For this review, take the finished solid that the model builds, in its own axes (mm). A direction names the side the tool comes from. Coordinates: 2 decimals unless noted, no trailing zeros. Loops run counter-clockwise (first coordinate to the right, second up) from the corner with the lowest first, then second, coordinate; pieces in that order, holes last. Notation, with made-up numbers: M -17,68 L 24,68 A11 cw 24,77 Z; hole C -15.75,-4 d1. An arc over 180 degrees is marked long. Put each result on its own line as item: value.
Autodesk Inventor part; units mm, degrees
ref_plane "YZ Plane" through (0, 0, 0) normal (1, 0, 0) x (0, 1, 0)
ref_plane "XZ Plane" through (0, 0, 0) normal (0, 1, 0) x (-1, 0, 0)
ref_plane "XY Plane" through (0, 0, 0) normal (0, 0, 1) x (1, 0, 0)
sketch "草图1" plane through (0, 0, 0) normal (0, 0, 1) x (1, 0, 0)
  line L0 (53.15, -38.15) -> (-53.15, -38.15)
  line L1 (-53.15, -38.15) -> (-53.15, 38.15)
  line L2 (-53.15, 38.15) -> (53.15, 38.15)
  line L3 (53.15, 38.15) -> (53.15, -38.15)
  line L4 (53.15, -38.15) -> (-53.15, 38.15) construction
  line L5 (-53.15, -38.15) -> (53.15, 38.15) construction
  point P0 (0, 0)
  dimension "d0" = 106.3
  dimension "d1" = 76.3
extrude "拉伸1" add sketch "草图1" along normal blind 3
sketch "草图4" plane through (0, 0, 3) normal (0, 0, 1) x (1, 0, 0)
  line L0 (24.8622, 25) -> (24.8622, -25) construction
  line L1 (21.8622, 25) -> (21.8622, -25)
  line L2 (27.8622, -25) -> (27.8622, 25)
  arc A0 (27.8622, 25) -> (21.8622, 25) centre (24.8622, 25) ccw
  arc A1 (21.8622, -25) -> (27.8622, -25) centre (24.8622, -25) ccw
  line L3 (-32.0429, 25) -> (-32.0429, -25) construction
  line L4 (-35.0429, 25) -> (-35.0429, -25)
  line L5 (-29.0429, -25) -> (-29.0429, 25)
  arc A2 (-29.0429, 25) -> (-35.0429, 25) centre (-32.0429, 25) ccw
  arc A3 (-35.0429, -25) -> (-29.0429, -25) centre (-32.0429, -25) ccw
  point P0 (0, 0)
  point P1 (24.8622, 0)
  point P2 (-32.0429, 0)
  dimension "d4" = 50
  dimension "d5" = 6
  dimension "d6" = 50
  dimension "d7" = 6
extrude "拉伸2" cut sketch "草图4" against normal blind 3
(1) Add section A-A (y = 17). Write out the cut boundary in (x, z).
Determined:
outline: M -53.15,0 L -35.04,0 L -35.04,3 L -53.15,3 Z; M -29.04,0 L 21.86,0 L 21.86,3 L -29.04,3 Z; M 27.86,0 L 53.15,0 L 53.15,3 L 27.86,3 Z
(2) Tool access review of faces 1 (the flat face through (-35.043, 0, 2)), 2 (the flat face through (-1, 1, 0)): name each direction out of +Z, -Z, +X, -X, +Y, -Y from which nothing blocks a thin tool from reaching the whole face with its end or side.
Determined:
face 1: +Z, -Z
face 2: -Z, +X, -X, +Y, -Y
(3) Add section B-B (x = 26.5). Write out the cut boundary in (y, z), plus the area to 3 significant figures.
Determined:
outline: M -38.15,0 L -27.51,0 L -27.51,3 L -38.15,3 Z; M 27.51,0 L 38.15,0 L 38.15,3 L 27.51,3 Z
area: 63.8 mm^2
(4) Draft analysis for pull direction Y (two halves, no side actions). For faces 3 (the cylindrical face through (-32, 28, 2)), 4 (the flat face through (-1, 38.15, 1)), 5 (the flat face through (1, -38.15, 1)), 6 (the flat face through (-53.15, -1, 1)), state which applies: +Y half, -Y half, draft (parallel to the pull), parting line (faces both ways), or undercut.
Determined:
face 3: undercut
face 4: +Y half
face 5: -Y half
face 6: draft
(5) Add section C-C (z = 2.25). Write out the cut boundary in (x, y), plus the area to 3 significant figures.
Determined:
outline: M -53.15,-38.15 L 53.15,-38.15 L 53.15,38.15 L -53.15,38.15 Z; hole M -35.04,-25 A3 ccw -29.04,-25 L -29.04,25 A3 ccw -35.04,25 Z; hole M 21.86,-25 A3 ccw 27.86,-25 L 27.86,25 A3 ccw 21.86,25 Z
area: 7,450 mm^2
(6) Wall thickness on line 1 along X through (y, z) = (2, 1.5); line 2 along X through (y, z) = (-26, 2.15); line 3 along Y through (x, z) = (23.5, 1.8): over which ranges is each line inside the solid? List them lowest first. Write a range as [from, to].
Determined:
line 1: x = [-53.15, -35.04], [-29.04, 21.86], [27.86, 53.15]
line 2: x = [-53.15, -34.87], [-29.21, 22.03], [27.69, 53.15]
line 3: y = [-38.15, -27.67], [27.67, 38.15]
